Autodesk Inventor part; units mm, degrees
ref_plane "YZ Plane" through (0, 0, 0) normal (1, 0, 0) x (0, 1, 0)
ref_plane "XZ Plane" through (0, 0, 0) normal (0, 1, 0) x (-1, 0, 0)
ref_plane "XY Plane" through (0, 0, 0) normal (0, 0, 1) x (1, 0, 0)
sketch "Sketch1" plane through (0, 0, 0) normal (0, 1, 0) x (-1, 0, 0)
  line L0 (72, -76) -> (-72, -76)
  line L1 (-72, -76) -> (-72, 76)
  line L2 (-72, 76) -> (72, 76)
  line L3 (72, 76) -> (72, -76)
  line L4 (72, -76) -> (-72, 76) construction
  line L5 (-72, -76) -> (72, 76) construction
  point P0 (0, 0)
  dimension "d3" = 152
  dimension "d4" = 144
extrude "Extrusion1" add sketch "Sketch1" along normal blind 10
sketch "Sketch2" plane through (0, 10, 0) normal (0, 1, 0) x (1, 0, 0)
  line L0 (-9.5175, -400.0105) -> (-9.5175, -295.6322)
  line L1 (-12.5175, -292.6322) -> (-116.9815, -292.6322)
  line L2 (-119.9815, -295.6322) -> (-119.9815, -400.0105)
  line L3 (-116.9815, -403.0105) -> (-12.5175, -403.0105)
  circle A0 centre (0.2505, -407.097) radius 1.7294
  circle A1 centre (-129.7495, -407.097) radius 1.7294
  circle A2 centre (-84.7495, -287.097) radius 1.7294
  line L4 (-18.5175, -301.6322) -> (-110.9815, -301.6322)
  line L5 (-18.5175, -394.0105) -> (-18.5175, -301.6322)
  line L6 (-110.9815, -301.6322) -> (-110.9815, -394.0105)
  line L7 (-110.9815, -394.0105) -> (-18.5175, -394.0105)
  line L8 (-12.5175, -298.6322) -> (-12.5175, -397.0105)
  line L9 (-15.5175, -400.0105) -> (-113.9815, -400.0105)
  line L10 (-116.9815, -397.0105) -> (-116.9815, -298.6322)
  line L11 (-113.9815, -295.6322) -> (-15.5175, -295.6322)
  arc A3 (-116.9815, -397.0105) -> (-113.9815, -400.0105) centre (-113.9815, -397.0105) ccw
  arc A4 (-119.9815, -400.0105) -> (-116.9815, -403.0105) centre (-116.9815, -400.0105) ccw
  arc A5 (-15.5175, -400.0105) -> (-12.5175, -397.0105) centre (-15.5175, -397.0105) ccw
  arc A6 (-12.5175, -403.0105) -> (-9.5175, -400.0105) centre (-12.5175, -400.0105) ccw
  arc A7 (-9.5175, -295.6322) -> (-12.5175, -292.6322) centre (-12.5175, -295.6322) ccw
  arc A8 (-12.5175, -298.6322) -> (-15.5175, -295.6322) centre (-15.5175, -298.6322) ccw
  arc A9 (-116.9815, -292.6322) -> (-119.9815, -295.6322) centre (-116.9815, -295.6322) ccw
  arc A10 (-113.9815, -295.6322) -> (-116.9815, -298.6322) centre (-113.9815, -298.6322) ccw
  line L12 (-46.232, -37.913) -> (46.232, -37.913)
  line L13 (46.232, -37.913) -> (46.232, 54.465)
  line L14 (46.232, 54.465) -> (-46.232, 54.465)
  line L15 (-46.232, 54.465) -> (-46.232, -37.913)
  line L16 (72, -76) -> (72, 76) construction
  line L17 (72, 76) -> (-72, 76) construction
  point P0 (0, 0)
  point P1 (-67.2495, -360.597)
  dimension "d7" = 9
  dimension "d8" = 9
  dimension "d9" = 9
  dimension "d10" = 9
  dimension "d11" = 3
  dimension "d12" = 3
  dimension "d13" = 92.378
  dimension "d14" = 92.464
  dimension "d15" = 25.768
  dimension "d16" = 21.535
  dimension "d19" = 144
  dimension "d20" = 152
extrude "Extrusion2" cut sketch "Sketch2" against normal blind 10 contours L15 L14 L13 L12
sketch "Sketch3" plane through (0, 10, 0) normal (0, 1, 0) x (1, 0, 0)
  line L0 (-46.232, 54.465) -> (46.232, 54.465) construction
  line L1 (72, -76) -> (72, 76) construction
  line L2 (-72, 76) -> (-72, -76) construction
  line L3 (-72, -76) -> (72, -76) construction
  line L4 (72, 76) -> (-72, 76) construction
  point P0 (0, 0)
  point P1 (0, 0)
  point P2 (-65, -6)
  point P3 (-65, 39)
  point P4 (-65, -51)
  point P5 (65, -6)
  point P6 (65, 39)
  point P7 (65, -51)
  point P8 (-20, 69)
  point P9 (20, 69)
  dimension "d21" = 45
  dimension "d22" = 45
  dimension "d23" = 45
  dimension "d24" = 45
  dimension "d25" = 14.535
  dimension "d26" = 14.535
  dimension "d27" = 40
  dimension "d28" = 52
  dimension "d29" = 7
  dimension "d30" = 7
  dimension "d31" = 7
  dimension "d32" = 7
  dimension "d33" = 7
  dimension "d34" = 25
  dimension "d36" = 25
hole "Hole1" at (-65, 10, 6) at (-65, 10, -39) at (-65, 10, 51) at (65, 10, 6) at (65, 10, -39) at (65, 10, 51) at (-20, 10, -69) at (20, 10, -69) direction (0, -1, 0) diameter 3.5 end through all
sketch "Sketch4" plane through (0, 10, 0) normal (0, 1, 0) x (1, 0, 0)
  line L0 (55.232, -43.913) -> (55.232, 60.465)
  line L1 (52.232, 63.465) -> (-52.232, 63.465)
  line L2 (-55.232, 60.465) -> (-55.232, -43.913)
  line L3 (-52.232, -46.913) -> (52.232, -46.913)
  circle A0 centre (502.0315, -140.3134) radius 1.7294
  circle A1 centre (372.0315, -140.3134) radius 1.7294
  circle A2 centre (417.0315, -20.3134) radius 1.7294
  line L4 (46.232, 54.465) -> (-46.232, 54.465)
  line L5 (46.232, -37.913) -> (46.232, 54.465)
  line L6 (-46.232, 54.465) -> (-46.232, -37.913)
  line L7 (-46.232, -37.913) -> (46.232, -37.913)
  line L8 (52.232, 57.465) -> (52.232, -40.913)
  line L9 (49.232, -43.913) -> (-49.232, -43.913)
  line L10 (-52.232, -40.913) -> (-52.232, 57.465)
  line L11 (-49.232, 60.465) -> (49.232, 60.465)
  arc A3 (-52.232, -40.913) -> (-49.232, -43.913) centre (-49.232, -40.913) ccw
  arc A4 (-55.232, -43.913) -> (-52.232, -46.913) centre (-52.232, -43.913) ccw
  arc A5 (49.232, -43.913) -> (52.232, -40.913) centre (49.232, -40.913) ccw
  arc A6 (52.232, -46.913) -> (55.232, -43.913) centre (52.232, -43.913) ccw
  arc A7 (55.232, 60.465) -> (52.232, 63.465) centre (52.232, 60.465) ccw
  arc A8 (52.232, 57.465) -> (49.232, 60.465) centre (49.232, 57.465) ccw
  arc A9 (-52.232, 63.465) -> (-55.232, 60.465) centre (-52.232, 60.465) ccw
  arc A10 (-49.232, 60.465) -> (-52.232, 57.465) centre (-49.232, 57.465) ccw
  line L12 (-46.232, 54.465) -> (46.232, 54.465)
  line L13 (46.232, -37.913) -> (-46.232, -37.913)
  line L14 (46.232, 54.465) -> (46.232, -37.913)
  line L15 (-46.232, -37.913) -> (-46.232, 54.465)
  point P0 (0, 0)
  point P1 (-14.6695, 0.7102)
  dimension "d44" = 9
  dimension "d45" = 9
  dimension "d46" = 9
  dimension "d47" = 9
  dimension "d48" = 3
  dimension "d49" = 3
  dimension "d51" = 0
  dimension "d52" = 0
  dimension "d53" = 0
  dimension "d54" = 0
extrude "Extrusion3" cut sketch "Sketch4" against normal blind 2.5 contours A6 L3 A4 L2 A9 L1 A7 L0
sketch "Sketch5" plane through (0, 10, 0) normal (0, 1, 0) x (1, 0, 0)
  line L0 (58.232, -49.913) -> (-58.232, -49.913)
  line L1 (-58.232, -49.913) -> (-58.232, 65.465)
  line L2 (-58.232, 65.465) -> (58.232, 65.465)
  line L3 (58.232, 65.465) -> (58.232, -49.913)
  line L4 (72, 76) -> (-72, 76)
  line L5 (-55.232, -43.913) -> (-55.232, 60.465)
  line L6 (55.232, 60.465) -> (55.232, -43.913)
  line L7 (52.232, -46.913) -> (-52.232, -46.913)
  line L8 (-52.232, 63.465) -> (52.232, 63.465)
  point P0 (0, 0)
  point P1 (58.232, 76)
  point P2 (-58.232, 76)
  dimension "d58" = 3
  dimension "d59" = 3
  dimension "d60" = 3
  dimension "d65" = 2
extrude "Extrusion4" cut sketch "Sketch5" against normal blind 3.1
extrude "Extrusion5" cut sketch "Sketch4" against normal blind 5.6 contours A6 L3 A4 L2 A9 L1 A7 L0
properties part number "Glass holder"
The listing builds one solid part. Answer for the finished solid, in the listing's coordinates (mm). A direction names the side the tool comes from. Coordinates: 2 decimals unless noted, no trailing zeros. Loops run counter-clockwise (first coordinate to the right, second up) from the corner with the lowest first, then second, coordinate; pieces in that order, holes last. Notation, with made-up numbers: (2, 31) - (11, 31) arc R33 ccw to (11, 65) - close; hole circle Ø6 at (11.5, 59). An arc over 180 degrees is marked (long way). Use a Markdown table: item, result. Add a question column.
1) The part is cut by section D-D, the plane z = 0. Give the vertices of the cut face in (x, y).
2) Find the intervals of material crossed by line 1 (X direction, y = 4, z = 6); line 2 (X direction, y = 5.75, z = 6); line 3 (Z direction, x = 65, y = 5.5), in increasing order.
3) The part is cut by section B-B, the plane z = -39. Give the vertices of the cut face in (x, y), and give its area (3 significant figures).
4) Given pin 1 (6 mm diameter, centred on x = -9, z = 48, fed in from -Y), flat-ended and moving along its own axis, determine where the tip first touches the part or whether it passes through.
5) The part is cut by section C-C, the plane y = 1.75. State how many separate pieces and enclosed holes the cut face has, and give its area (3 significant figures).
6) For faces 4 (the flat face through (1, 3, -54.465)), 5 (the flat face through (1, 5, 76)), 6 (the flat face through (-4, 4.4, 45)), determine the directions among +Z, -Z, +X, -X, +Y, -Y from which every point of the face is accessible in a straight line to the end or side of a thin tool.
7) The mould has two halves that part along X. Classify faces 1 (the flat face through (1, 0, 52)), 2 (the flat face through (72, 5, -1)), 3 (the flat face through (-1, 3, 37.913)): released by +X, released by -X, zero draft, split by the parting line, or undercut.
8) The part is cut by section A-A, the plane x = -20. Give the vertices of the cut face in (y, z) (3 decimals).
Here are the results:
| question | item | result |
|---|---|---|
| 1 | outline | (-72, 0) - (-46.23, 0) - (-46.23, 6.9) - (-52.23, 6.9) - (-52.23, 4.4) - (-55.23, 4.4) - (-55.23, 6.9) - (-58.23, 6.9) - (-58.23, 10) - (-72, 10) - close; (46.23, 0) - (72, 0) - (72, 10) - (58.23, 10) - (58.23, 6.9) - (55.23, 6.9) - (55.23, 4.4) - (52.23, 4.4) - (52.23, 6.9) - (46.23, 6.9) - close |
| 2 | line 1 | x = -72 to -66.75, -63.25 to -46.23, 46.23 to 63.25, 66.75 to 72 |
| 2 | line 2 | x = -72 to -66.75, -63.25 to -55.23, -52.23 to -46.23, 46.23 to 52.23, 55.23 to 63.25, 66.75 to 72 |
| 2 | line 3 | z = -76 to -40.75, -37.25 to 4.25, 7.75 to 49.25, 52.75 to 76 |
| 3 | outline | (-72, 0) - (-66.75, 0) - (-66.75, 10) - (-72, 10) - close; (-63.25, 0) - (-46.23, 0) - (-46.23, 6.9) - (-52.23, 6.9) - (-52.23, 4.4) - (-55.23, 4.4) - (-55.23, 6.9) - (-58.23, 6.9) - (-58.23, 10) - (-63.25, 10) - close; (46.23, 0) - (63.25, 0) - (63.25, 10) - (58.23, 10) - (58.23, 6.9) - (55.23, 6.9) - (55.23, 4.4) - (52.23, 4.4) - (52.23, 6.9) - (46.23, 6.9) - close; (66.75, 0) - (72, 0) - (72, 10) - (66.75, 10) - close |
| 3 | area | 356 mm^2 |
| 4 | pin 1 | stops at y = 0 |
| 5 | separate pieces | 1 |
| 5 | enclosed holes | 9 |
| 5 | area | 13,300 mm^2 |
| 6 | face 4 | +Y, -Y |
| 6 | face 5 | +Z, +X, -X, +Y, -Y |
| 6 | face 6 | +Y |
| 7 | face 1 | zero draft |
| 7 | face 2 | released by +X |
| 7 | face 3 | undercut |
| 8 | outline | (0, -76) - (10, -76) - (10, -70.75) - (0, -70.75) - close; (0, -67.25) - (10, -67.25) - (10, -65.465) - (6.9, -65.465) - (6.9, -63.465) - (4.4, -63.465) - (4.4, -60.465) - (6.9, -60.465) - (6.9, -54.465) - (0, -54.465) - close; (0, 37.913) - (6.9, 37.913) - (6.9, 43.913) - (4.4, 43.913) - (4.4, 46.913) - (6.9, 46.913) - (6.9, 49.913) - (10, 49.913) - (10, 76) - (0, 76) - close |
